Source: CAD feature listing. Evaluate the final solid. Frame: model axes, mm. Face numbers are marked on the shaded views. A direction names the side the tool comes from. Coordinates: 2 decimals unless noted, no trailing zeros. Loops run counter-clockwise (first coordinate to the right, second up) from the corner with the lowest first, then second, coordinate; pieces in that order, holes last. Notation, with made-up numbers: (-25.5, 19) - (32.5, 19) arc R24 cw to (32.5, 51) - close; hole circle Ø3 at (69, -5.75). An arc over 180 degrees is marked (long way). Use one line per item in the form item = value. Start each with the question number.
from build123d import *

# Parameters (mm, degrees)
BOSS_EXTRUDE1_DEPTH                                 = 9.525
CUT_EXTRUDE7_DEPTH                                  = 0.2
CUT_EXTRUDE8_DEPTH                                  = 0.2
CBORE_FOR_8_BINDING_HEAD_MACHINE_SCREW4_D           = 4.4958
CBORE_FOR_8_BINDING_HEAD_MACHINE_SCREW4_DEPTH       = 12.024265282
CBORE_FOR_8_BINDING_HEAD_MACHINE_SCREW4_CBORE_D     = 6.985
CBORE_FOR_8_BINDING_HEAD_MACHINE_SCREW4_CBORE_DEPTH = 10.024265282
CHAMFER4_SIZE                                       = 0.5


with BuildPart() as part:
    # Sketch32 → Boss-Extrude1 (new body)
    with BuildSketch(Plane(origin=(0, 4.7625, 0), x_dir=(1, 0, 0), z_dir=(0, 1, 0))):
        with BuildLine():
            Line((14.278748413, -0.5), (7.190320252, -0.5))
            Line((7.190320252, -0.5), (3.739497694, -6.477))
            Line((3.739497694, -6.477), (-3.739497694, -6.477))
            Line((-3.739497694, -6.477), (-7.190320252, -0.5))
            Line((-7.190320252, -0.5), (-14.278748413, -0.5))
            ThreePointArc((-14.278748413, -0.5), (0, -14.2875), (14.278748413, -0.5))
        make_face()
    extrude(amount=-BOSS_EXTRUDE1_DEPTH)

    # Sketch37 → Cut-Revolve4 (revolve, cut)
    with BuildSketch(Plane(origin=(0, 0, 0), x_dir=(-0.99776158, 0, -0.06687174), z_dir=(0.06687174, 0, -0.99776158))):
        Polygon((0, -4.7625), (0, -3.7625), (-6.477, -3.7625), (-7.477, -4.7625), align=None)
    revolve(axis=Axis((0, -4.7625, 0), (0, 1, 0)), mode=Mode.SUBTRACT)

    # Sketch43 → Cut-Revolve5 (revolve, cut)
    with BuildSketch(Plane(origin=(0, 0, 0), x_dir=(-0.99776158, 0, 0.06687174), z_dir=(-0.06687174, 0, -0.99776158))):
        Polygon((0, 4.7625), (0, 3.7625), (6.477, 3.7625), (7.477, 4.7625), align=None)
    revolve(axis=Axis((0, 4.7625, 0), (0, -1, 0)), mode=Mode.SUBTRACT)

    # Sketch48 → Cut-Extrude7 (cut)
    with BuildSketch(Plane(origin=(0, 4.7625, 0), x_dir=(1, 0, 0), z_dir=(0, 1, 0))):
        with BuildLine():
            Line((14.278748413, -0.5), (9.987492178, -0.5))
            ThreePointArc((9.987492178, -0.5), (0, -10), (-9.987492178, -0.5))
            Line((-9.987492178, -0.5), (-14.278748413, -0.5))
            ThreePointArc((-14.278748413, -0.5), (0, -14.2875), (14.278748413, -0.5))
        make_face()
    extrude(amount=-CUT_EXTRUDE7_DEPTH, mode=Mode.SUBTRACT)

    # Sketch49 → Cut-Extrude8 (cut)
    with BuildSketch(Plane.XZ.offset(4.7625)):
        with BuildLine():
            Line((9.987492178, 0.5), (14.278748413, 0.5))
            ThreePointArc((14.278748413, 0.5), (0, 14.2875), (-14.278748413, 0.5))
            Line((-14.278748413, 0.5), (-9.987492178, 0.5))
            ThreePointArc((-9.987492178, 0.5), (0, 10), (9.987492178, 0.5))
        make_face()
    extrude(amount=-CUT_EXTRUDE8_DEPTH, mode=Mode.SUBTRACT)

    # CBORE for #8 Binding Head Machine Screw4
    with Locations(Plane.XY.offset(12.524265282)):
        with Locations((-10.368210259, 0), (10.368210259, 0)):
            CounterBoreHole(CBORE_FOR_8_BINDING_HEAD_MACHINE_SCREW4_D / 2, CBORE_FOR_8_BINDING_HEAD_MACHINE_SCREW4_CBORE_D / 2, CBORE_FOR_8_BINDING_HEAD_MACHINE_SCREW4_CBORE_DEPTH, depth=CBORE_FOR_8_BINDING_HEAD_MACHINE_SCREW4_DEPTH)

    # Chamfer4
    chamfer4_edges = [part.edges().sort_by_distance(p)[0] for p in [
        (0, 4.5625, 14.2875),
        (0, -4.5625, 14.2875),
    ]]
    chamfer(chamfer4_edges, length=CHAMFER4_SIZE)


solid = part.part
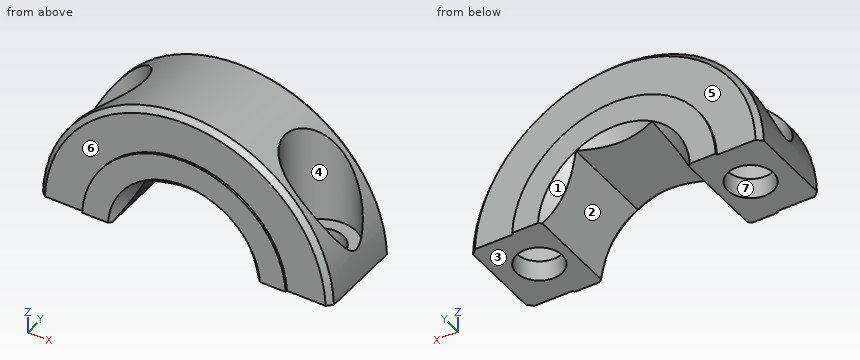
(1) Access query for the marked faces 1, 2, 3 and 4. Directions: +Z, -Z, +X, -X, +Y, -Y. A direction counts if a zero-diameter tool reaches every point of the face in a straight line with its end or side. Return the directions, or none.
(2) Cut plane C-C, the plane z = 1.75. State how many separate pieces and enclosed holes the cut face has, plus the area to 3 significant figures.
(3) Contact query for flat-ended pins moving along their axis: pin 1 (4 mm diameter, centred on x = 10.37, y = 0, fed in from +Z); pin 2 (3.5 mm diameter, centred on x = -11, y = 1, fed in from +Z); pin 3 (2 mm diameter, centred on x = 6.5, z = 10, fed in from -Y); pin 4 (3.5 mm diameter, centred on x = 1.5, y = -1, fed in from -Z). Output: stop coordinate, or through.
(4) Mould query, pull axis Y, two halves, no side actions, for the marked faces 5, 6 and 7. Classes: +Y half, -Y half, draft (parallel to the pull), parting line (faces both ways), or undercut.
(5) Cut plane A-A, the plane x = 0. Output: boundary loops of the cut face in (y, z).
(6) Cut plane D-D, the plane y = -3. Output: boundary loops of the cut face in (x, z) (1 decimal).
(7) Cut plane B-B, the plane y = 0. Output: boundary loops of the cut face in (x, z) (1 decimal), plus the area to 3 significant figures.
(8) Material intervals for line 1 (X direction, y = 1.75, z = 4); line 2 (Y direction, x = 6.25, z = 8.25); line 3 (X direction, y = 4.5, z = 6.25), sorted ascending.
Recorded:
q1.face_1 = -Z, +Y
q1.face_2 = -Z, +Y, -Y
q1.face_3 = -Z, +X, -X, +Y, -Y
q1.face_4 = +Z
q2.separate_pieces = 2
q2.enclosed_holes = 2
q2.area = 110 mm²
q3.pin_1 = through
q3.pin_2 = 2.5
q3.pin_3 = -4.56
q3.pin_4 = 6.48
q4.face_5 = +Y half
q4.face_6 = -Y half
q4.face_7 = undercut
q5.outline = (-4.76, 7.48) - (-3.76, 6.48) - (3.76, 6.48) - (4.76, 7.48) - (4.76, 10) - (4.56, 10) - (4.56, 13.79) - (4.06, 14.29) - (-4.06, 14.29) - (-4.56, 13.79) - (-4.56, 10) - (-4.76, 10) - close
q6.outline = (-14.3, 0.5) - (-7.2, 0.5) - (-3.7, 6.5) - (3.7, 6.5) - (7.2, 0.5) - (14.3, 0.5) arc R14.3 ccw to (12.2, 7.5) - (12.2, 2.5) - (8.6, 2.5) - (8.6, 11.4) arc R14.3 ccw to (-8.6, 11.4) - (-8.6, 2.5) - (-12.2, 2.5) - (-12.2, 7.5) arc R14.3 ccw to start
q7.outline = (-14.3, 0.5) - (-12.6, 0.5) - (-12.6, 2.5) - (-13.9, 2.5) - (-13.9, 3.5) arc R14.3 ccw to start; (-8.1, 0.5) - (-7.2, 0.5) - (-3.7, 6.5) - (3.7, 6.5) - (7.2, 0.5) - (8.1, 0.5) - (8.1, 2.5) - (6.9, 2.5) - (6.9, 12.5) arc R14.3 ccw to (-6.9, 12.5) - (-6.9, 2.5) - (-8.1, 2.5) - close; (12.6, 0.5) - (14.3, 0.5) arc R14.3 ccw to (13.9, 3.5) - (13.9, 2.5) - (12.6, 2.5) - close
q7.area = 128 mm²
q8.line_1 = -13.72 to -13.39, -7.35 to -5.17, 5.17 to 7.35, 13.39 to 13.72
q8.line_2 = -4.56 to 4.56
q8.line_3 = -12.36 to -3.87, 3.87 to 12.36
